Design review of the part built by this model. Coordinates are the model's own, in mm. A direction names the side the tool comes from. Coordinates: 2 decimals unless noted, no trailing zeros. Write each loop counter-clockwise with the first axis right and the second up, starting at its lowest first coordinate (ties: lowest second). Pieces come first, ordered by that corner, then holes. Notation, with made-up numbers: (-16, -36.75) - (26, -36.75) arc R18 cw to (26, -30.75) - close; hole circle Ø1 at (8.25, 27). An arc over 180 degrees is marked (long way). Answer as a JSON object with one key per item and string values.
```python
from build123d import *

# Parameters (mm, degrees)
F0_W     = 25
F0_H     = 30
F1_DEPTH = 2
F2_R     = 1.5
F3_DEPTH = 2.001
F4_W     = 25
F4_H     = 6.1
F5_DEPTH = 0.7
F6_SIZE  = 10
F7_R     = 7


with BuildPart() as f1:
    # F0 (on Top) → F1 (new body)
    with BuildSketch(Plane.XY):
        Rectangle(F0_W, F0_H)
    extrude(amount=F1_DEPTH)

    # F2 (on face) → F3 (cut, through all)
    with BuildSketch(Plane.XY.offset(2)):
        with Locations((-2, -12)):
            Circle(F2_R)
        with Locations((4.5, -1.5)):
            Circle(F2_R)
        with Locations((4.5, 8.5)):
            Circle(F2_R)
    extrude(amount=-F3_DEPTH, mode=Mode.SUBTRACT)

    # F4 (on face) → F5 (cut)
    with BuildSketch(Plane.XY.offset(2)):
        with Locations((0, -6.95)):
            Rectangle(F4_W, F4_H)
    extrude(amount=-F5_DEPTH, mode=Mode.SUBTRACT)

    # F6
    f6_edges = [f1.edges().sort_by_distance(p)[0] for p in [
        (-12.5, 15, 1),
    ]]
    chamfer(f6_edges, length=F6_SIZE)

    # F7
    f7_edges = [f1.edges().sort_by_distance(p)[0] for p in [
        (-12.5, 5, 1),
        (-2.5, 15, 1),
        (12.5, 15, 1),
    ]]
    fillet(f7_edges, radius=F7_R)


solid = f1.part
```
(1) For pin 1 (1.8 mm diameter, centred on x = -4, y = -8, fed in from +Z), flat-tipped, find the tip position at first contact; note if it passes through.
Solved:
{"pin 1": "stops at z = 1.3"}
(2) Tool access review of faces 5 (the face through (10.4, 13, 1)), 6 (the face through (0, -7, 1.3)): name each direction out of +Z, -Z, +X, -X, +Y, -Y from which nothing blocks a thin tool from reaching the whole face with its end or side.
Solved:
{"face 5": "+Z, -Z, +X, +Y", "face 6": "+Z, +X, -X"}
(3) To check wall thickness, follow line 1 (Y direction, x = 4.5, z = 1.35); line 2 (Y direction, x = 4.5, z = 1.25); line 3 (Y direction, x = -2.25, z = 1.5). State the ranges of each line that lie inside material, in increasing order. Write a range as from..to.
Solved:
{"line 1": "y = -15..-10, -3.9..-3, 0..7, 10..15", "line 2": "y = -15..-3, 0..7, 10..15", "line 3": "y = -15..-13.48, -10.52..-10, -3.9..14.48"}
(4) Take a section at A-A, the plane z = 1.6. Write out the cut boundary in (x, y).
Solved:
{"outline": "(-12.5, -15) - (12.5, -15) - (12.5, -10) - (-12.5, -10) - close; (-12.5, -3.9) - (12.5, -3.9) - (12.5, 8) arc R7 ccw to (5.5, 15) - (0.4, 15) arc R7 ccw to (-4.55, 12.95) - (-10.45, 7.05) arc R7 ccw to (-12.5, 2.1) - close; hole circle Ø3 at (-2, -12); hole circle Ø3 at (4.5, -1.5); hole circle Ø3 at (4.5, 8.5)"}
(5) The part is to be moulded in two halves that separate along X. For faces 1 (the face through (5.19, 7.17, 1.01)), 2 (the face through (-2.315, 14.452, 1.014)), 3 (the face through (5.886, -2.075, 1.014)), 4 (the face through (0, -15, 1)), say which applies: pulls with the +X half, pulls with the -X half, needs draft (parallel to the pull), parting line crosses it, or undercut.
Solved:
{"face 1": "undercut", "face 2": "pulls with the -X half", "face 3": "undercut", "face 4": "needs draft"}
(6) Take a section at D-D, the plane x = -6. Write out the cut boundary in (y, z), and give its area (3 significant figures).
Solved:
{"outline": "(-15, 0) - (11.5, 0) - (11.5, 2) - (-3.9, 2) - (-3.9, 1.3) - (-10, 1.3) - (-10, 2) - (-15, 2) - close", "area": "48.7 mm^2"}
(7) Take a section at B-B, the plane y = -12. Write out the cut boundary in (x, z), and give its area (3 significant figures).
Solved:
{"outline": "(-12.5, 0) - (-3.5, 0) - (-3.5, 2) - (-12.5, 2) - close; (-0.5, 0) - (12.5, 0) - (12.5, 2) - (-0.5, 2) - close", "area": "44.0 mm^2"}
(8) Take a section at C-C, the plane x = 4.5. Write out the cut boundary in (y, z).
Solved:
{"outline": "(-15, 0) - (-3, 0) - (-3, 2) - (-3.9, 2) - (-3.9, 1.3) - (-10, 1.3) - (-10, 2) - (-15, 2) - close; (0, 0) - (7, 0) - (7, 2) - (0, 2) - close; (10, 0) - (15, 0) - (15, 2) - (10, 2) - close"}
